Source: CAD feature listing. Evaluate the final solid. Frame: model axes, mm. A direction names the side the tool comes from. Round coordinates to 2 decimals unless told otherwise and drop trailing zeros. Write each loop counter-clockwise with the first axis right and the second up, starting at its lowest first coordinate (ties: lowest second). Pieces come first, ordered by that corner, then holes. Notation, with made-up numbers: M 48.25,16.5 L 89.25,16.5 A17 ccw 89.25,32.5 Z; hole C -25,82.25 d11. An arc over 180 degrees is marked long. Put each result on its own line as item: value. Start each with the question number.
```python
from build123d import *

# Parameters (mm, degrees)
SKETCH_1_R          = 7.5
EXTRUDE_1_DEPTH     = 12.6
SKETCH_2_W          = 11.291748881
SKETCH_2_H          = 5
EXTRUDE_2_DEPTH     = 32.6
SKETCH_3_R          = 1.5
CUT_EXTRUDE_1_DEPTH = 45.373528145
FILLET_1_R          = 3
SKETCH_4_W          = 3
SKETCH_4_H          = 15
EXTRUDE_3_DEPTH     = 20
SKETCH_5_R          = 1.3
CUT_EXTRUDE_2_DEPTH = 46.967488511
SKETCH_6_W          = 36.00279958
SKETCH_6_H          = 34.73430716
CUT_EXTRUDE_3_DEPTH = 46.967488511
SKETCH_7_R          = 1.5
EXTRUDE_4_DEPTH     = 3
SKETCH_8_R          = 1.5
CUT_EXTRUDE_4_DEPTH = 45.373528145
SKETCH_9_R          = 3
CUT_EXTRUDE_5_DEPTH = 4


with BuildPart() as part:
    # 草图1 → 凸台-拉伸1 (new body)
    with BuildSketch(Plane.XY):
        with BuildLine():
            Line((-10.956194261, 6.017624724), (-22.5, -15))
            Line((-22.5, -15), (-22.5, -20))
            Line((-22.5, -20), (22.5, -20))
            Line((22.5, -20), (22.5, -15))
            Line((22.5, -15), (10.956194261, 6.017624724))
            ThreePointArc((10.956194261, 6.017624724), (0, 12.5), (-10.956194261, 6.017624724))
        make_face()
        Circle(SKETCH_1_R, mode=Mode.SUBTRACT)
    extrude(amount=EXTRUDE_1_DEPTH)

    # 草图2 → 凸台-拉伸2 (add)
    with BuildSketch(Plane.XY):
        with Locations((-16.854125559, -17.5)):
            Rectangle(SKETCH_2_W, SKETCH_2_H)
        with Locations((16.854125559, -17.5)):
            Rectangle(SKETCH_2_W, SKETCH_2_H)
    extrude(amount=EXTRUDE_2_DEPTH)

    # 草图3 → 切除-拉伸1 (cut, through all)
    with BuildSketch(Plane(origin=(0, 0, 0), x_dir=(1, 0, 0), z_dir=(0, 1, 0))):
        with Locations(Location((-17.5, -26.3, 0), (0, 0, 270))):
            Circle(SKETCH_3_R)
        with Locations((17.5, -26.3)):
            Circle(SKETCH_3_R)
    extrude(amount=-CUT_EXTRUDE_1_DEPTH, mode=Mode.SUBTRACT)

    # 圆角1
    fillet_1_edges = [part.edges().sort_by_distance(p)[0] for p in [
        (-22.5, -17.5, 32.6),
        (-11.208251119, -17.5, 32.6),
        (11.208251119, -17.5, 32.6),
    ]]
    fillet(fillet_1_edges, radius=FILLET_1_R)

    # 草图4 → 凸台-拉伸3 (add, through all)
    with BuildSketch(Plane(origin=(0, 0, 0), x_dir=(1, 0, 0), z_dir=(0, 1, 0))):
        with Locations((24, -25.1)):
            Rectangle(SKETCH_4_W, SKETCH_4_H)
    extrude(amount=-EXTRUDE_3_DEPTH)

    # 草图5 → 切除-拉伸2 (cut, through all)
    with BuildSketch(Plane(origin=(0, 0, 0), x_dir=(0, 0, -1), z_dir=(1, 0, 0))):
        with Locations(Location((-25.1, -3, 0), (0, 0, 180))):
            Circle(SKETCH_5_R)
        with Locations(Location((-25.1, -12.5, 0), (0, 0, 180))):
            Circle(SKETCH_5_R)
    extrude(amount=CUT_EXTRUDE_2_DEPTH, mode=Mode.SUBTRACT)

    # 草图6 → 切除-拉伸3 (cut, through all)
    with BuildSketch(Plane(origin=(0, 0, 0), x_dir=(0, 0, -1), z_dir=(1, 0, 0))):
        with Locations((-15.759025291, -4.011160204)):
            Rectangle(SKETCH_6_W, SKETCH_6_H)
    extrude(amount=CUT_EXTRUDE_3_DEPTH, mode=Mode.SUBTRACT)

    # 草图7 → 凸台-拉伸4 (add)
    with BuildSketch(Plane(origin=(0, 0, 0), x_dir=(0, 0, -1), z_dir=(1, 0, 0))):
        with BuildLine():
            Line((-9.3, 7.5), (-9.3, 12.5))
            Line((-9.3, 12.5), (-9.3, 15.5))
            ThreePointArc((-9.3, 15.5), (-6.3, 18.5), (-3.3, 15.5))
            Line((-3.3, 15.5), (-3.3, 7.5))
            Line((-3.3, 7.5), (-9.3, 7.5))
        make_face()
        with Locations((-6.3, 15.5)):
            Circle(SKETCH_7_R, mode=Mode.SUBTRACT)
    extrude(amount=-EXTRUDE_4_DEPTH)

    # 草图8 → 切除-拉伸4 (cut, through all)
    with BuildSketch(Plane(origin=(0, 0, 0), x_dir=(0, 0, -1), z_dir=(1, 0, 0))):
        with Locations((-6.3, -12.5)):
            Circle(SKETCH_8_R)
    extrude(amount=-CUT_EXTRUDE_4_DEPTH, mode=Mode.SUBTRACT)

    # 草图9 → 切除-拉伸5 (cut)
    with BuildSketch(Plane(origin=(-22.5, 0, 0), x_dir=(0, 0, -1), z_dir=(1, 0, 0))):
        with Locations(Location((-6.3, -12.5, 0), (0, 0, 236.442690238))):
            Circle(SKETCH_9_R)
    extrude(amount=CUT_EXTRUDE_5_DEPTH, mode=Mode.SUBTRACT)


solid = part.part
```
(1) Section query C-C (x = -12.75). Return loops of the section in (y, z), and give its area (3 significant figures).
(2) Pull-direction query (Z, two-part tool) for faces 1 (the flat face through (-17, -15, 22)), 2 (the cylindrical face through (-9.12, -13.964, 6.625)), 3 (the cylindrical face through (-1.5, 18.5, 6.4)); classes: +Z half, -Z half, draft (parallel to the pull), parting line (faces both ways), or undercut.
(3) Access query for faces 4 (the flat face through (-3, 14, 7)), 5 (the cylindrical face through (-20.084, -15.383, 7.131)), 6 (the cylindrical face through (-7.5, 0.16, 6.21)). Directions: +Z, -Z, +X, -X, +Y, -Y. A direction counts if a zero-diameter tool reaches every point of the face in a straight line with its end or side. Return the directions, or none.
(4) Section query B-B (y = -12.5). Return loops of the section in (x, z), and give its area (3 significant figures).
(5) Ray query, line 1 along X through (y, z) = (-17.95, 26.3); line 2 along Y through (x, z) = (-2.05, 6.3); line 3 along Z through (x, y) = (-19.95, -12.5). Return the intervals inside material, ascending.
(6) Contact query for flat-ended pins moving along their axis: P1, Ø3.5, axis at x = -18.5, z = 22.5, coming from the +Y side; P2, Ø5, axis at y = -12.5, z = 6.3, coming from the -X side; P3, Ø2.5, axis at x = -1, y = 14, coming from the +Z side; P4, Ø10, axis at x = -6, z = 19.5, coming from the +Y side. Output: stop coordinate, or through.
(7) Section query D-D (z = 10.5). Return loops of the section in (x, y), and give its area (3 significant figures).
(8) Section query A-A (z = 6.3). Return loops of the section in (x, y), and give its area (3 significant figures).
Entries:
1. outline: M -20,0 L 2.75,0 L 2.75,12.6 L -15,12.6 L -15,32.22 L -20,32.22 Z; hole C -12.5,6.3 d3
1. area: 378 mm2
2. face 1: draft
2. face 2: undercut
2. face 3: parting line
3. face 4: +Z, -Z, -X, +Y
3. face 5: -X
3. face 6: +Z, -Z, +X
4. outline: M -21.13,0 L 0,0 L 0,4.8 L -18.5,4.8 L -18.5,3.3 L -21.13,3.3 Z; M -21.13,9.3 L -18.5,9.3 L -18.5,7.8 L 0,7.8 L 0,12.6 L -21.13,12.6 Z
4. area: 195 mm2
5. line 1: -22.5 to -19, -16 to -11.21
5. line 2: -20 to -14, -11 to -7.21, 7.21 to 14, 17 to 18.5
5. line 3: 0 to 3.3, 9.3 to 12.6
6. P1: y = -15
6. P2: x = -18.5
6. P3: z = 9.3
6. P4: through
7. outline: M -22.5,-20 L 0,-20 L 0,-7.5 A7.5 cw 0,7.5 L 0,12.5 A12.5 ccw -10.96,6.02 L -22.5,-15 Z
7. area: 426 mm2
8. outline: M -22.5,-20 L 0,-20 L 0,-14 L -18.5,-14 L -18.5,-15.5 L -22.5,-15.5 Z; M -19.48,-9.5 L -18.5,-9.5 L -18.5,-11 L 0,-11 L 0,-7.5 A7.5 cw 0,7.5 L 0,14 L -3,14 L -3,12.13 A12.5 ccw -10.96,6.02 Z; M -3,17 L 0,17 L 0,18.5 L -3,18.5 Z
8. area: 364 mm2
